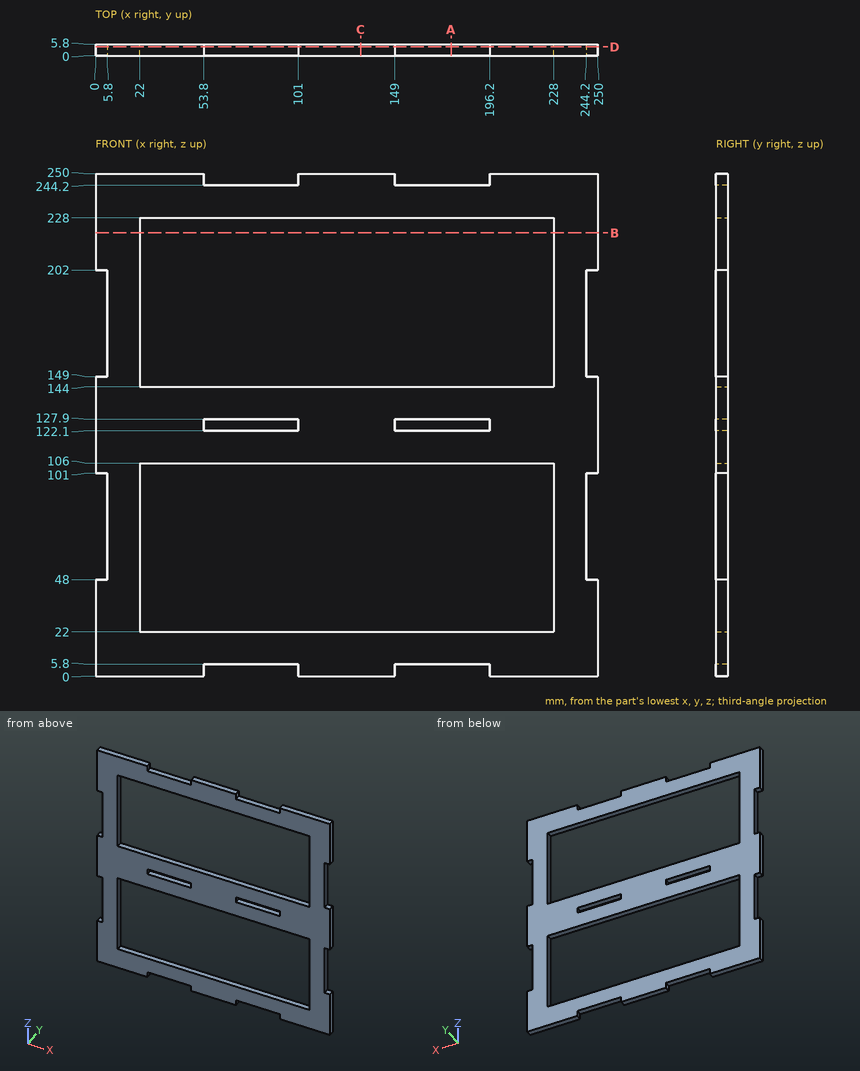
Drawing for the job (mm, zero at the part's lowest x, y, z). Round coordinates to 2 decimals unless told otherwise and drop trailing zeros. Loops run counter-clockwise (first coordinate to the right, second up) from the corner with the lowest first, then second, coordinate; pieces in that order, holes last. Notation, with made-up numbers: (77.25, -24) - (109.25, -24) arc R21 ccw to (109.25, 3) - close; hole circle Ø1 at (69, -23). An arc over 180 degrees is marked (long way). Return JSON: item names as keys, results as strings. Group by question number.
Q1. Band-saw the part on D-D on y = 4.4. Give the number of separate pieces and of enclosed holes in the cut face, plus the area to 3 significant figures.
Q2. Flat gauge pins, fed straight in: pin 1 Ø3 at (y, z) = (2, 167) entering from +X; pin 2 Ø3 at (x, y) = (175.5, 2) entering from +Z; pin 3 Ø3 at (y, z) = (3, 60.5) entering from -X. Where does each tip first touch, or does it go through?
Q3. Band-saw the part on A-A on x = 177. Give the cut face in (y, z).
Q4. Band-saw the part on B-B on z = 220.5. Give the cut face in (x, y).
Q5. Drill centre lines: line 1 along Z through (x, y) = (155, 2.85); line 2 along Z through (x, y) = (36.5, 3); line 3 along X through (y, z) = (2.5, 124). Where is each one in solid material? Low to high. Write a range as [from, to].
Q6. Band-saw the part on C-C on x = 132. Give the cut face in (y, z), plus the area to 3 significant figures.
Solutions:
{
 "1": {"separate pieces": "1", "enclosed holes": "4", "area": "25,000 mm^2"},
 "2": {"pin 1": "stops at x = 244.2", "pin 2": "stops at z = 244.2", "pin 3": "stops at x = 5.8"},
 "3": {"outline": "(0, 5.8) - (5.8, 5.8) - (5.8, 22) - (0, 22) - close; (0, 106) - (5.8, 106) - (5.8, 122.1) - (0, 122.1) - close; (0, 127.9) - (5.8, 127.9) - (5.8, 144) - (0, 144) - close; (0, 228) - (5.8, 228) - (5.8, 244.2) - (0, 244.2) - close"},
 "4": {"outline": "(0, 0) - (22, 0) - (22, 5.8) - (0, 5.8) - close; (228, 0) - (250, 0) - (250, 5.8) - (228, 5.8) - close"},
 "5": {"line 1": "z = [5.8, 22], [106, 122.1], [127.9, 144], [228, 244.2]", "line 2": "z = [0, 22], [106, 144], [228, 250]", "line 3": "x = [0, 53.8], [101, 149], [196.2, 250]"},
 "6": {"outline": "(0, 0) - (5.8, 0) - (5.8, 22) - (0, 22) - close; (0, 106) - (5.8, 106) - (5.8, 144) - (0, 144) - close; (0, 228) - (5.8, 228) - (5.8, 250) - (0, 250) - close", "area": "476 mm^2"}
}
